Check sheet for the modelled part. Datum: model origin and axes. Units: mm. Round coordinates to 2 decimals unless told otherwise and drop trailing zeros. Loops run counter-clockwise (first coordinate to the right, second up) from the corner with the lowest first, then second, coordinate; pieces in that order, holes last. Notation, with made-up numbers: (-31.5, 71.5) - (17.5, 71.5) arc R32 ccw to (17.5, 106.5) - close; hole circle Ø2 at (35, 62.25). An arc over 180 degrees is marked (long way). Answer in a Markdown table with one row per item. Add a question column.
(1) Thickness scan on line 1 along X through (y, z) = (130, -18.5); line 2 along Y through (x, z) = (112, -40); line 3 along Y through (x, z) = (180, -51). Record the ranges inside material, lowest first.
(2) Cross-section at C-C on z = -40. Enter the section's corners in (x, y), then the cut area to 3 significant figures.
(3) Cross-section at D-D on y = 130. Enter the section's corners in (x, z).
(4) Mould release check, pull along X, two halves, no side actions. Record for faces 1 (the flat face through (250, 128, -39)), 2 (the cylindrical face through (123.25, 54.297, -24.015)), 3 (the cylindrical face through (170.493, 131.248, -40.56)): +X half, -X half, draft (parallel to the pull), parting line (faces both ways), or undercut.
(5) Cross-section at B-B on y = 215. Enter the section's corners in (x, z), then the cut area to 3 significant figures.
(6) Cross-section at A-A on x = 180. Enter the section's corners in (y, z).
Autodesk Inventor part; units mm, degrees
ref_plane "YZ Plane" through (0, 0, 0) normal (1, 0, 0) x (0, 1, 0)
ref_plane "XZ Plane" through (0, 0, 0) normal (0, 1, 0) x (-1, 0, 0)
ref_plane "XY Plane" through (0, 0, 0) normal (0, 0, 1) x (1, 0, 0)
sketch "Sketch1" plane through (0, 0, 0) normal (0, 0, 1) x (1, 0, 0)
  line L0 (0, 0) -> (250, 0)
  line L1 (250, 0) -> (250, 260)
  line L2 (250, 260) -> (0, 260)
  line L3 (0, 260) -> (0, 0)
  dimension "d0" = 250
  dimension "d1" = 260
extrude "Extrusion1" add sketch "Sketch1" against normal blind 80
sketch "Sketch2" plane through (250, 0, 0) normal (1, 0, 0) x (0, 0, -1)
  line L0 (0, 0) -> (0, 260)
  line L1 (0, 260) -> (80, 260)
  point P0 (40, 205)
  point P1 (40, 55)
  dimension "d4" = 40
  dimension "d5" = 40
  dimension "d6" = 150
  dimension "d7" = 55
hole "Hole1" at (250, 205, -40) at (250, 55, -40) direction (-1, 0, 0) diameter 32 end through all
sketch "Sketch3" plane through (0, 0, 0) normal (0, 0, 1) x (1, 0, 0)
  line L0 (0, 0) -> (250, 0)
  line L1 (250, 260) -> (0, 260)
  line L2 (0, 260) -> (0, 0)
  line L3 (250, 0) -> (250, 260)
  point P0 (70, 130)
  point P1 (180, 130)
  dimension "d16" = 130
  dimension "d17" = 130
  dimension "d18" = 70
  dimension "d19" = 70
hole "Hole2" at (70, 130, 0) at (180, 130, 0) direction (0, 0, -1) diameter 19.177 end through all
properties part number "Soporte barras"
Answers:
| question | item | result |
|---|---|---|
| 1 | line 1 | x = 0 to 60.41, 79.59 to 170.41, 189.59 to 250 |
| 1 | line 2 | y = 0 to 39, 71 to 189, 221 to 260 |
| 1 | line 3 | y = 0 to 43.38, 66.62 to 120.41, 139.59 to 193.38, 216.62 to 260 |
| 2 | outline | (0, 0) - (250, 0) - (250, 39) - (0, 39) - close; (0, 71) - (250, 71) - (250, 189) - (0, 189) - close; (0, 221) - (250, 221) - (250, 260) - (0, 260) - close; hole circle Ø19.18 at (70, 130); hole circle Ø19.18 at (180, 130) |
| 2 | area | 48,400 mm^2 |
| 3 | outline | (0, -80) - (60.41, -80) - (60.41, 0) - (0, 0) - close; (79.59, -80) - (170.41, -80) - (170.41, 0) - (79.59, 0) - close; (189.59, -80) - (250, -80) - (250, 0) - (189.59, 0) - close |
| 4 | face 1 | +X half |
| 4 | face 2 | draft |
| 4 | face 3 | undercut |
| 5 | outline | (0, -80) - (250, -80) - (250, -52.49) - (0, -52.49) - close; (0, -27.51) - (250, -27.51) - (250, 0) - (0, 0) - close |
| 5 | area | 13,800 mm^2 |
| 6 | outline | (0, -80) - (120.41, -80) - (120.41, 0) - (0, 0) - close; (139.59, -80) - (260, -80) - (260, 0) - (139.59, 0) - close; hole circle Ø32 at (55, -40); hole circle Ø32 at (205, -40) |
